Autodesk Fusion 360 part; units mm, degrees
sketch "Sketch1" plane through (0, 0, 0) normal (0, 0, 1) x (1, 0, 0)
  circle A0 centre (0, 0) radius 6.6
  circle A1 centre (0, 0) radius 9.6
  dimension "d1" = 3
  dimension "d2" = 13.2
extrude "Extrude1" add sketch "Sketch1" along normal blind 13
extrude "Extrude2" add sketch "Sketch1" against normal blind 2 contours A0 | A1
fillet "Fillet1" radius 3 1 edges at (-8.9503, 3.4715, -2)
Geometry: final body of the model. Coordinates: model frame, mm. A direction names the side the tool comes from. Round coordinates to 2 decimals unless told otherwise and drop trailing zeros. Order: outer loops, then holes, each group sorted by start corner. A loop starts at its lowest first (then second) coordinate and runs counter-clockwise, first axis right, second up. Notation, with made-up numbers: M 16.25,-10.5 L 33.25,-10.5 A13 cw 33.25,-5.5 Z; hole C 38.25,68 d2. An arc over 180 degrees is marked long. One line per item, written item: value.
(1) Cut plane A-A (z = 5). Return the cut outline in (x, y).
Result sheet:
outline: C 0,0 d19.2; hole C 0,0 d13.2
(2) Pull-direction query (Y, two-part tool) for faces 3 (the flat face through (-7, -2, 13)), 4 (the cylindrical face through (-1.25, -9.52, 6.92)), 5 (the cylindrical face through (-4.864, -4.461, 6.409)); classes: pulls with the +Y half, pulls with the -Y half, needs draft (parallel to the pull), parting line crosses it, or undercut.
Result sheet:
face 3: needs draft
face 4: parting line crosses it
face 5: undercut
(3) Line query: probe 1 along Y at (x, z) = (0, 6); probe 2 along Z at (x, y) = (-2.5, -5.25); probe 3 along Y at (x, z) = (2.5, 10.5). Output: solid intervals per line, ascending. Write a range as [from, to].
Result sheet:
probe 1: [-9.6, -6.6], [6.6, 9.6]
probe 2: [-2, 0]
probe 3: [-9.27, -6.11], [6.11, 9.27]
(4) Pin query (flat end, axial travel): P1, Ø1, axis at x = -5, y = -1.5, coming from the +Z side; P2, Ø2, axis at y = 2, z = 2, coming from the +X side; P3, Ø3, axis at x = -3, z = 5.5, coming from the +Y side. Return the tip coordinate at first contact, or that it passes through.
Result sheet:
P1: z = 0
P2: x = 9.55
P3: y = 9.48
(5) Reachability of faces 1 (the flat face through (0, 0, -2)), 2 (the flat face through (0, 0, 0)) from +Z, -Z, +X, -X, +Y, -Y: full face, straight path, thin tool, end or side. Return the list, or none.
Result sheet:
face 1: -Z, +X, -X, +Y, -Y
face 2: +Z
